from build123d import *

# Parameters (mm, degrees)
BOSS_EXTRUDE1_DEPTH      = 3
BOSS_EXTRUDE1_DEPTH_BACK = 3
SKETCH1_W                = 100
SKETCH1_H                = 60
SKETCH2_W                = 4.95
SKETCH2_H                = 2.9
CUT_EXTRUDE1_DEPTH       = 11
DRAFT1_ANGLE             = 1
SKETCH3_W                = 96
SKETCH3_H                = 52
CUT_EXTRUDE2_DEPTH       = 2
FILLET1_R                = 2
SKETCH4_R                = 2.5
CUT_EXTRUDE3_DEPTH       = 59.446556785
CHAMFER1_SIZE            = 0.5
SKETCH5_R                = 1.882569545
CUT_EXTRUDE4_DEPTH       = 0.5


with BuildPart() as part:
    # Sketch1 → Boss-Extrude1 (new, two sides: drawn at the far end of the back side and taken through both)
    with BuildSketch(Plane.XY.offset(-BOSS_EXTRUDE1_DEPTH_BACK)):
        Rectangle(SKETCH1_W, SKETCH1_H)
    extrude(amount=BOSS_EXTRUDE1_DEPTH + BOSS_EXTRUDE1_DEPTH_BACK)

    # Sketch2 → Cut-Extrude1 (cut)
    with BuildSketch(Plane.XZ.offset(30)):
        with Locations((0, 0.3)):
            Rectangle(SKETCH2_W, SKETCH2_H)
    extrude(amount=-CUT_EXTRUDE1_DEPTH, mode=Mode.SUBTRACT)

    # Draft1
    draft1_faces = [part.faces().sort_by_distance(p)[0] for p in [
        (-2.475, -24.5, 0.3),
        (2.475, -24.5, 0.3),
    ]]
    draft(draft1_faces, Plane(origin=(-50, -30, -3), x_dir=(-1, 0, 0), z_dir=(0, -1, 0)), DRAFT1_ANGLE)

    # Sketch3 → Cut-Extrude2 (cut)
    with BuildSketch(Plane.XY.offset(3)):
        with Locations((0, 2)):
            Rectangle(SKETCH3_W, SKETCH3_H)
    extrude(amount=-CUT_EXTRUDE2_DEPTH, mode=Mode.SUBTRACT)

    # Fillet1
    fillet1_edges = [part.edges().sort_by_distance(p)[0] for p in [
        (-50, 30, 0),
        (50, 30, 0),
        (50, -30, 0),
        (-50, -30, 0),
    ]]
    fillet(fillet1_edges, radius=FILLET1_R)

    # Sketch4 → Cut-Extrude3 (cut, through all)
    with BuildSketch(Plane.XY.offset(1)):
        with Locations((-43.453932042, 22.8)):
            Circle(SKETCH4_R)
        with Locations((-43.453932042, -19)):
            Circle(SKETCH4_R)
        with Locations((39.832771039, -19)):
            Circle(SKETCH4_R)
        with Locations((39.832771039, 22.8)):
            Circle(SKETCH4_R)
    extrude(amount=-CUT_EXTRUDE3_DEPTH, mode=Mode.SUBTRACT)

    # Chamfer1
    chamfer1_edges = [part.edges().sort_by_distance(p)[0] for p in [
        (-48, 2, 3),
        (0, -24, 3),
        (48, 2, 3),
        (0, 28, 3),
    ]]
    chamfer(chamfer1_edges, length=CHAMFER1_SIZE)

    # Sketch5 → Cut-Extrude4 (cut)
    with BuildSketch(Plane.XY.offset(3)):
        with Locations((0, -27.056295937)):
            Circle(SKETCH5_R)
    extrude(amount=-CUT_EXTRUDE4_DEPTH, mode=Mode.SUBTRACT)


solid = part.part
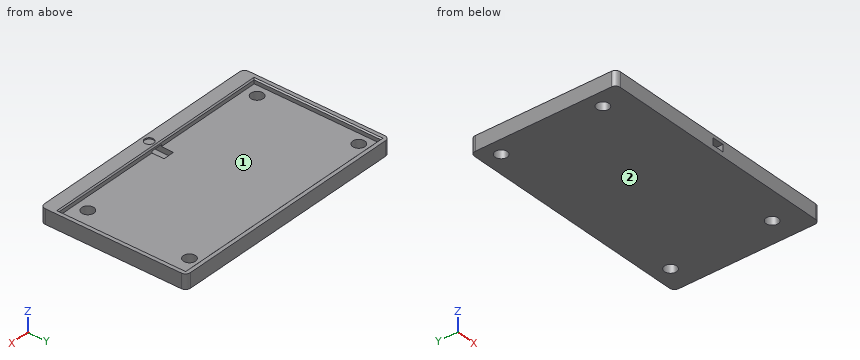
Geometry check sheet. Reference: the model listing, model coordinates, mm. Face numbers are marked on the shaded views. Give positions to 0.01 mm unless a question says otherwise; leave off trailing zeros. Order: outer loops, then holes, each group sorted by start corner. A loop starts at its lowest first (then second) coordinate and runs counter-clockwise, first axis right, second up. Notation, with made-up numbers: M 40,-25 L 52,-25 A14 ccw 52,-1 Z; hole C 53,-37.75 d5. An arc over 180 degrees is marked long. Use a Markdown table: item, result.
Item 1: Section check B-B (x = 0). Record the cut outline in (y, z), and give its area (3 significant figures).
Answers follow:
| item | result |
|---|---|
| outline | M -30,-3 L 30,-3 L 30,3 L 28.5,3 L 28,2.5 L 28,1 L -19,1 L -19,-1.15 L -30,-1.15 Z; M -30,1.75 L -24,1.75 L -24,2.5 L -24.5,3 L -25.17,3 L -25.17,2.5 L -28.94,2.5 L -28.94,3 L -30,3 Z |
| area | 226 mm2 |
Item 2: Section check C-C (y = 9.5). Record the cut outline in (x, z).
Answers follow:
| item | result |
|---|---|
| outline | M -50,-3 L 50,-3 L 50,3 L 48.5,3 L 48,2.5 L 48,1 L -48,1 L -48,2.5 L -48.5,3 L -50,3 Z |
Item 3: Draft check along Y on the marked faces 1 and 2. Enter one of: +Y half, -Y half, draft (parallel to the pull), parting line (faces both ways), or undercut.
Answers follow:
| item | result |
|---|---|
| face 1 | undercut |
| face 2 | draft |
Item 4: Section check D-D (y = -20.5). Record the cut outline in (x, z), and give its area (3 significant figures).
Answers follow:
| item | result |
|---|---|
| outline | M -50,-3 L -45.45,-3 L -45.45,1 L -48,1 L -48,2.5 L -48.5,3 L -50,3 Z; M -41.45,-3 L 37.83,-3 L 37.83,1 L 2.31,1 L 2.31,-1.15 L -2.31,-1.15 L -2.31,1 L -41.45,1 Z; M 41.83,-3 L 50,-3 L 50,3 L 48.5,3 L 48,2.5 L 48,1 L 41.83,1 Z |
| area | 366 mm2 |
Item 5: Material ranges on line 1 along Y through (x, z) = (-2, 2); line 2 along X through (y, z) = (-20.5, -2); line 3 along X through (y, z) = (22, -0.75), recorded low to high.
Answers follow:
| item | result |
|---|---|
| line 1 | y = -30 to -24, 28 to 30 |
| line 2 | x = -50 to -45.45, -41.45 to 37.83, 41.83 to 50 |
| line 3 | x = -50 to -45.82, -41.09 to 37.46, 42.2 to 50 |
Item 6: Depth check by flat-ended pin: P1, Ø8, axis at x = 39.83, y = 22.8, coming from the +Z side; P2, Ø4.5, axis at x = -43.45, y = 22.8, coming from the +Z side; P3, Ø1.1, axis at x = 1, z = -0.5, coming from the -Y side; P4, Ø2.5, axis at x = 0, y = -27.06, coming from the +Z side. Enter the tip coordinate at first touch or a pass-through.
Answers follow:
| item | result |
|---|---|
| P1 | stops at z = 1 |
| P2 | passes through |
| P3 | stops at y = -19 |
| P4 | stops at z = 2.5 |
Item 7: Section check A-A (y = 22.8). Record the cut outline in (x, z).
Answers follow:
| item | result |
|---|---|
| outline | M -50,-3 L -45.95,-3 L -45.95,1 L -48,1 L -48,2.5 L -48.5,3 L -50,3 Z; M -40.95,-3 L 37.33,-3 L 37.33,1 L -40.95,1 Z; M 42.33,-3 L 50,-3 L 50,3 L 48.5,3 L 48,2.5 L 48,1 L 42.33,1 Z |
